Verification items for the finished model (mm, model axes). A direction names the side the tool comes from. Round coordinates to 2 decimals unless told otherwise and drop trailing zeros. Loops run counter-clockwise (first coordinate to the right, second up) from the corner with the lowest first, then second, coordinate; pieces in that order, holes last.
from build123d import *

# Parameters (mm, degrees)
F0_R     = 7.5
F1_DEPTH = 50
F2_R     = 1
F4_D     = 3.3
F4_DEPTH = 14.1
F4_TIP   = 0.9914200214
F6_D     = 3.3
F6_DEPTH = 14.1
F6_TIP   = 0.9914200214


with BuildPart() as f1:
    # F0 (on Top) → F1 (new body)
    with BuildSketch(Plane.XY):
        Circle(F0_R)
    extrude(amount=F1_DEPTH)

    # F2
    f2_edges = [f1.edges().sort_by_distance(p)[0] for p in [
        (-7.5, 0, 50),
        (-7.5, 0, 0),
    ]]
    fillet(f2_edges, radius=F2_R)

    # F4
    with Locations(Plane.XY.offset(50)):
        with Locations((0, 0)):
            Hole(F4_D / 2, depth=F4_DEPTH)
            with Locations((0, 0, -(F4_DEPTH + F4_TIP / 2))):  # 118° drill point
                Cone(0, F4_D / 2, F4_TIP, mode=Mode.SUBTRACT)

    # F6
    with Locations(Plane(origin=(0, 0, 0), x_dir=(1, 0, 0), z_dir=(0, 0, -1))):
        with Locations((0, 0)):
            Hole(F6_D / 2, depth=F6_DEPTH)
            with Locations((0, 0, -(F6_DEPTH + F6_TIP / 2))):  # 118° drill point
                Cone(0, F6_D / 2, F6_TIP, mode=Mode.SUBTRACT)


solid = f1.part
1. Tool access check on faces 1 (the face through (1.216, 1.115, 42.851)), 2 (the face through (0.3, -0.1, 14.9)). Record the directions out of +Z, -Z, +X, -X, +Y, -Y that give a thin tool (end or side, any length) a straight path to the whole face; none if there is none.
2. Section check B-B (z = 19). Enter the section's corners in (x, y).
3. Release check for a two-part mould opening along Y. For faces 3 (the face through (1.216, -1.115, 7.149)), 4 (the face through (-7.493, 0.33, 24.664)), 5 (the face through (1.4, -1.4, 50)) record: released by +Y, released by -Y, zero draft, split by the parting line, or undercut.
4. Gauge pin test, flat ends, axial feed: P1, Ø1.5, axis at x = -3, z = 9, coming from the -Y side; P2, Ø3, axis at y = -2.5, z = 20.5, coming from the -X side; P3, Ø3, axis at x = 0, y = 0, coming from the -Z side. Record the tip position at first contact, or that the pin passes through.
5. Scan lines: L1, parallel to Y at x = 0, z = 47; L2, parallel to X at y = 1.5, z = 44; L3, parallel to X at y = 5.75, z = 10.5. Record each from-to range of solid material in increasing order.
6. Section check A-A (z = 44). Enter the section's corners in (x, y).
Taken from the geometry:
1. face 1: +Z
1. face 2: -Z
2. outline: circle Ø15 at (0, 0)
3. face 3: undercut
3. face 4: split by the parting line
3. face 5: zero draft
4. P1: stops at y = -7.15
4. P2: stops at x = -7.43
4. P3: stops at z = 14.19
5. L1: y = -7.5 to -1.65, 1.65 to 7.5
5. L2: x = -7.35 to -0.69, 0.69 to 7.35
5. L3: x = -4.82 to 4.82
6. outline: circle Ø15 at (0, 0); hole circle Ø3.3 at (0, 0)
